The listing builds one solid part. Answer for the finished solid, in the listing's coordinates (mm). A direction names the side the tool comes from. Give positions to 0.01 mm unless a question says otherwise; leave off trailing zeros. Loops run counter-clockwise (first coordinate to the right, second up) from the corner with the lowest first, then second, coordinate; pieces in that order, holes last. Notation, with made-up numbers: M 37,10 L 41,10 A20 cw 41,30 Z; hole C 3,38.25 d4. An arc over 180 degrees is marked long. Use one line per item in the form item = value. Start each with the question number.
1. For faces 5 (the face through (107.644, -102, 15)), 6 (the face through (58.83, -118.05, 15.28)), 7 (the face through (77.3, -160.65, 60.73)), determine the directions among +Z, -Z, +X, -X, +Y, -Y from which every point of the face is accessible in a straight line to the end or side of a thin tool.
2. The mould has two halves that part along Y. Classify faces 1 (the face through (88.06, -117.18, -29.58)), 2 (the face through (82, -164, 82)), 3 (the face through (88.37, -117.222, 15.283)), 4 (the face through (56.442, -98, 15)): released by +Y, released by -Y, zero draft, split by the parting line, or undercut.
3. The part is cut by section B-B (z = 24). Write down the section's boundary in (x, y) (1 decimal), and give its area (3 significant figures).
4. The part is cut by section D-D (z = -34). Write down the section's boundary in (x, y), and give its area (3 significant figures).
5. The part is cut by section C-C (z = 52.5). Write down the section's boundary in (x, y), and give its area (3 significant figures).
6. Straight lines are drawn through the part: line 1 (Z direction, x = 87.5, y = -197); line 2 (Y direction, x = 81, z = -34.5); line 3 (X direction, y = -199, z = -14). For each, find the intervals that lie inside material, in ascending order. Write a range as from..to.
7. Each of these flat-tipped pins is pushed along its axis until it touches: pin 1 Ø1.5 at (y, z) = (-196, 29) entering from -X; pin 2 Ø2 at (x, z) = (69.5, -34.5) entering from -Y; pin 3 Ø3 at (x, z) = (63, 19) entering from +Y. Where does it stop, or does it pass through?
8. The part is cut by section A-A (y = -99.5). Write down the section's boundary in (x, z).
Autodesk Inventor part; units mm, degrees
ref_plane "YZ Plane" through (0, 0, 0) normal (1, 0, 0) x (0, 1, 0)
ref_plane "XZ Plane" through (0, 0, 0) normal (0, 1, 0) x (-1, 0, 0)
ref_plane "XY Plane" through (0, 0, 0) normal (0, 0, 1) x (1, 0, 0)
sketch "Boceto1" plane through (0, 0, 0) normal (0, 0, 1) x (1, 0, 0)
  line L0 (0, 0) -> (176.0622, 0) construction
  line L1 (176.0622, 0) -> (176.0622, -234.7497) construction
  line L2 (176.0622, -234.7497) -> (0, -234.7497) construction
  line L3 (0, -234.7497) -> (0, 0) construction
  circle A0 centre (60.6994, -75.2554) radius 7
  line L4 (60.9494, -90.2533) -> (60.9494, -105.0535)
  line L5 (60.9494, -105.0535) -> (60.9494, -107.7044)
  line L6 (60.9494, -107.7044) -> (64.462, -107.7044)
  line L7 (64.462, -107.7044) -> (78.6909, -116.9211)
  arc A1 (62.497, -121.017) -> (111.2784, -126.8512) centre (82.0598, -164.3014) ccw
  line L8 (75.685, -75.9112) -> (111.2784, -89.6384)
  line L9 (111.2784, -89.6384) -> (111.2784, -91.0916)
  line L10 (111.2784, -91.0916) -> (111.2784, -115.9371)
  line L11 (111.2784, -115.9371) -> (114.0242, -115.9371)
  line L12 (114.0242, -115.9371) -> (114.0242, -119.5079)
  line L13 (114.0242, -119.5079) -> (111.2784, -126.8512)
  line L14 (75.0889, -79.491) -> (107.6439, -92.9034)
  line L15 (107.6439, -92.9034) -> (107.6439, -107.7044)
  line L16 (107.6439, -107.7044) -> (98.0464, -119.5725)
  line L17 (62.497, -121.017) -> (55.0669, -115.0084)
  line L18 (55.0669, -115.0084) -> (55.0669, -107.7044)
  line L19 (55.0669, -107.7044) -> (56.4416, -106.0045)
  line L20 (56.4416, -106.0045) -> (56.4416, -89.6384)
  arc A2 (75.0889, -79.491) -> (75.685, -75.9112) centre (60.6994, -75.2554) ccw construction
  arc A3 (60.9494, -90.2533) -> (75.0889, -79.491) centre (60.6994, -75.2554) ccw
  arc A4 (56.4416, -89.6384) -> (60.9494, -90.2533) centre (60.6994, -75.2554) ccw construction
  arc A5 (75.685, -75.9112) -> (56.4416, -89.6384) centre (60.6994, -75.2554) ccw
  arc A6 (78.6909, -116.9211) -> (62.497, -121.017) centre (82.0598, -164.3014) ccw construction
  arc A7 (111.2784, -126.8512) -> (98.0464, -119.5725) centre (82.0598, -164.3014) ccw construction
  arc A8 (98.0464, -119.5725) -> (78.6909, -116.9211) centre (82.0598, -164.3014) ccw
  dimension "d2" = 14
  dimension "d5" = 95
  dimension "d9" = 30
extrude "Extrusión1" add sketch "Boceto1" along normal blind 31
sketch "Boceto2" plane through (0, 0, 31) normal (0, 0, 1) x (1, 0, 0)
  arc A0 (62.497, -121.017) -> (111.2784, -126.8512) centre (82.0598, -164.3014) ccw
  circle A1 centre (82.0598, -164.3014) radius 47.5
  point P0 (0, 0)
  point P1 (62.497, -121.017)
extrude "Extrusión2" add sketch "Boceto2" along normal blind 11
sketch "Boceto3" plane through (0, 0, 0) normal (0, 0, -1) x (-1, 0, 0)
  arc A0 (-111.2784, -126.8512) -> (-62.497, -121.017) centre (-82.0598, -164.3014) ccw
  circle A1 centre (-82.0598, -164.3014) radius 47.5
  point P0 (0, 0)
extrude "Extrusión3" add sketch "Boceto3" along normal blind 70
fillet "Empalme1" radius 10 1 edges at (101.6226, -207.5859, -70)
fillet "Empalme2" radius 2 1 edges at (52.8411, -201.7517, 42)
sketch "Boceto4" plane through (82.0598, -164.3014, 42) normal (0, 0, 1) x (1, 0, 0)
  circle A0 centre (0, 0) radius 6
  point P0 (-82.0598, 164.3014)
  dimension "d32" = 12
extrude "Extrusión4" add sketch "Boceto4" along normal blind 40
chamfer "Chaflán1" distance 2 angle 45 1 edges at (76.0598, -164.3014, 82)
fillet "Empalme3" radius 5 2 edges at (111.2784, -89.6384, 15.5) (107.6439, -92.9034, 15.5)
properties part number "motor2"
Derived:
q1.face_5 = +Z, -Z
q1.face_6 = +Z, -Z, -X
q1.face_7 = +Z
q2.face_1 = released by +Y
q2.face_2 = zero draft
q2.face_3 = undercut
q2.face_4 = undercut
q3.outline = M 55.1,-115 L 62.5,-121 A47.5 ccw long 111.3,-126.9 L 114,-119.5 L 114,-115.9 L 111.3,-115.9 L 111.3,-93.1 A5 ccw 108.1,-88.4 L 75.7,-75.9 A15 ccw long 56.4,-89.6 L 56.4,-106 L 55.1,-107.7 Z; hole C 60.7,-75.3 d14; hole M 60.9,-107.7 L 64.5,-107.7 L 78.7,-116.9 A47.5 cw 98,-119.6 L 107.6,-107.7 L 107.6,-96.3 A5 ccw 104.5,-91.6 L 75.1,-79.5 A15 cw 60.9,-90.3 Z
q3.area = 8,270 mm2
q4.outline = M 62.5,-121.02 A47.5 ccw long 111.28,-126.85 A47.5 ccw Z
q4.area = 7,090 mm2
q5.outline = C 82.06,-164.3 d12
q5.area = 113 mm2
q6.line_1 = -70..42
q6.line_2 = -211.79..-116.81
q6.line_3 = 49.62..114.5
q7.pin_1 = 46.03
q7.pin_2 = -210.37
q7.pin_3 = -60.28
q8.outline = M 56.44,0 L 60.95,0 L 60.95,31 L 56.44,31 Z; M 107.64,0 L 111.28,0 L 111.28,31 L 107.64,31 Z
